Geometry: final body of the model. Coordinates: model frame, mm. A direction names the side the tool comes from. Give positions to 0.01 mm unless a question says otherwise; leave off trailing zeros. Use one line per item in the form item = value.
from build123d import *

# Parameters (mm, degrees)
F0_W     = 250
F0_H     = 500
F1_DEPTH = 860
F2_R     = 25
F2_R_2   = 6.5
F3_DEPTH = 25
F4_R     = 6.5
F5_DEPTH = 25


with BuildPart() as f1:
    # F0 (on Top) → F1 (new body)
    with BuildSketch(Plane.XY):
        with Locations((4.553568, 192.676917)):
            Rectangle(F0_W, F0_H)
    extrude(amount=F1_DEPTH)

    # F2 (on face) → F3 (cut)
    with BuildSketch(Plane.XY.offset(860)):
        with Locations((4.553568, 372.676917)):
            Circle(F2_R)
        with Locations((4.553568, -7.323083)):
            Circle(F2_R_2)
    extrude(amount=-F3_DEPTH, mode=Mode.SUBTRACT)

    # F4 (on face) → F5 (cut)
    with BuildSketch(Plane(origin=(0, 0, 0), x_dir=(1, 0, 0), z_dir=(0, 0, -1))):
        with Locations((-35.446432, -12.676917)):
            Circle(F4_R)
    extrude(amount=-F5_DEPTH, mode=Mode.SUBTRACT)


solid = f1.part
(1) Contact query for a flat-ended pin moving along its axis: pin 1 Ø15 at (x, y) = (-6.5, 372.5) entering from +Z. Output: stop coordinate, or through.
Computed values:
pin_1 = 835
(2) Reachability of faces 1 (the face through (4, 373, 835)), 2 (the face through (3, 442.677, 424)) from +Z, -Z, +X, -X, +Y, -Y: full face, straight path, thin tool, end or side. Return the list, or none.
Computed values:
face_1 = +Z
face_2 = +Z, -Z, +X, -X, +Y
(3) Pull-direction query (Y, two-part tool) for faces 3 (the face through (3, 196, 0)), 4 (the face through (1.299, 397.464, 847.675)), 5 (the face through (3, -57.323, 424)); classes: released by +Y, released by -Y, zero draft, split by the parting line, or undercut.
Computed values:
face_3 = zero draft
face_4 = undercut
face_5 = released by -Y
